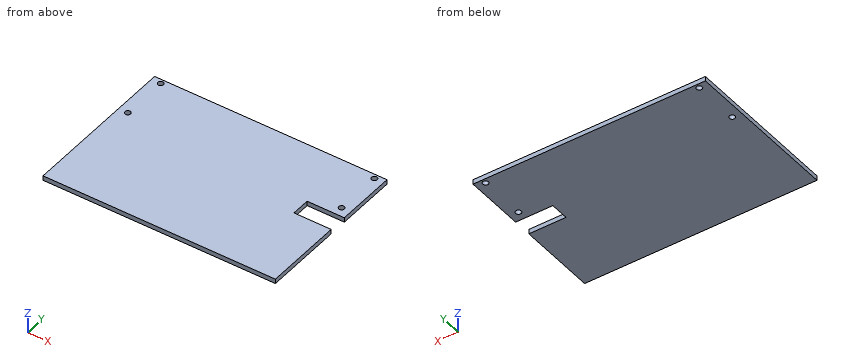
from build123d import *

# Parameters (mm, degrees)
ESQUISSE1_W             = 250
ESQUISSE1_H             = 170
ESQUISSE1_R             = 3
BOSS_EXTRU_1_DEPTH      = 5
ESQUISSE4_W             = 40
ESQUISSE4_H             = 20
ENL_V_MAT_EXTRU_1_DEPTH = 10


with BuildPart() as part:
    # Esquisse1 → Boss.-Extru.1 (new body)
    with BuildSketch(Plane.XY):
        with Locations((125, -85)):
            Rectangle(ESQUISSE1_W, ESQUISSE1_H)
        with Locations((10, -55)):
            Circle(ESQUISSE1_R, mode=Mode.SUBTRACT)
        with Locations((10, -5)):
            Circle(ESQUISSE1_R, mode=Mode.SUBTRACT)
        with Locations(Location((240, -55, 0), (0, 0, 180))):
            Circle(ESQUISSE1_R, mode=Mode.SUBTRACT)
        with Locations(Location((240, -5, 0), (0, 0, 180))):
            Circle(ESQUISSE1_R, mode=Mode.SUBTRACT)
    extrude(amount=BOSS_EXTRU_1_DEPTH)

    # Esquisse4 → Enlèv. mat.-Extru.1 (cut)
    with BuildSketch(Plane.XY.offset(5)):
        with Locations((230, -75)):
            Rectangle(ESQUISSE4_W, ESQUISSE4_H)
    extrude(amount=-ENL_V_MAT_EXTRU_1_DEPTH, mode=Mode.SUBTRACT)


solid = part.part
For this review, take the finished solid that the model builds, in its own axes (mm). Give positions to 0.01 mm unless a question says otherwise; leave off trailing zeros. Order: outer loops, then holes, each group sorted by start corner. A loop starts at its lowest first (then second) coordinate and runs counter-clockwise, first axis right, second up. Notation, with made-up numbers: (1.5, 49) - (27.5, 49) arc R24 cw to (27.5, 65) - close; hole circle Ø6 at (70, -6). An arc over 180 degrees is marked (long way). Answer as a JSON object with one key per item and string values. Group by question number.
Item 1: Take a section at C-C on z = 2.2. Give the boundary of the cut face in (x, y).
Item 2: Take a section at D-D on x = 10. Give the boundary of the cut face in (y, z), and give its area (3 significant figures).
Item 3: Take a section at B-B on y = -5. Give the boundary of the cut face in (x, z), and give its area (3 significant figures).
Item 4: Wall thickness on line 1 along Y through (x, z) = (10, 1.05); line 2 along Y through (x, z) = (240, 3.75); line 3 along Y through (x, z) = (212.5, 2.8): over which ranges is each line inside the solid? List them lowest first.
Item 5: Take a section at A-A on x = 220.5. Give the boundary of the cut face in (y, z).
Reported:
{
 "1": {"outline": "(0, -170) - (250, -170) - (250, -85) - (210, -85) - (210, -65) - (250, -65) - (250, 0) - (0, 0) - close; hole circle Ø6 at (10, -55); hole circle Ø6 at (10, -5); hole circle Ø6 at (240, -55); hole circle Ø6 at (240, -5)"},
 "2": {"outline": "(-170, 0) - (-58, 0) - (-58, 5) - (-170, 5) - close; (-52, 0) - (-8, 0) - (-8, 5) - (-52, 5) - close; (-2, 0) - (0, 0) - (0, 5) - (-2, 5) - close", "area": "790 mm^2"},
 "3": {"outline": "(0, 0) - (7, 0) - (7, 5) - (0, 5) - close; (13, 0) - (237, 0) - (237, 5) - (13, 5) - close; (243, 0) - (250, 0) - (250, 5) - (243, 5) - close", "area": "1,190 mm^2"},
 "4": {"line 1": "-170 to -58, -52 to -8, -2 to 0", "line 2": "-170 to -85, -65 to -58, -52 to -8, -2 to 0", "line 3": "-170 to -85, -65 to 0"},
 "5": {"outline": "(-170, 0) - (-85, 0) - (-85, 5) - (-170, 5) - close; (-65, 0) - (0, 0) - (0, 5) - (-65, 5) - close"}
}
